Design review of the part built by this model. Coordinates are the model's own, in mm. A direction names the side the tool comes from. Coordinates: 2 decimals unless noted, no trailing zeros. Write each loop counter-clockwise with the first axis right and the second up, starting at its lowest first coordinate (ties: lowest second). Pieces come first, ordered by that corner, then holes.
Q1. To check wall thickness, follow probe 1 along X at (y, z) = (-20, -19.5); probe 2 along Z at (x, y) = (39, -14.75); probe 3 along Y at (x, z) = (41, -9.75). State the ranges of each line that lie inside material, in increasing order.
Q2. Add section D-D, the plane z = -6.25. Give the boundary of the cut face in (x, y).
Q3. Add section C-C, the plane y = -5.25. Give the boundary of the cut face in (x, z), plus the area to 3 significant figures.
Q4. Add section B-B, the plane z = -14.5. Give the boundary of the cut face in (x, y).
Q5. Clearance check with flat-ended pins moving along their axes: pin 1 Ø3 at (x, z) = (41.5, -11.5) entering from -Y; pin 2 Ø6.5 at (x, y) = (46.5, -16.5) entering from -Z; pin 3 Ø3 at (x, z) = (41.5, -11.5) entering from +Y. State where each tip first meets the part, or that it passes through.
Q6. Add section A-A, the plane y = -13.5. Give the boundary of the cut face in (x, z), plus the area to 3 significant figures.
Q7. Machinability: for faces 1 (the face through (44, -6.903, -13)), 2 (the face through (44, -14, -7.729)), 3 (the face through (44, -20.663, -13)), 4 (the face through (44, -14, -17.984)), 5 (the face through (18, 0, -14)), which of the approach directions +Z, -Z, +X, -X, +Y, -Y give a long, thin tool a straight path to every point of the face, cutting with its end or side? Answer none if there is none.
from build123d import *

# Parameters (mm, degrees)
F0_W     = 37.3699069023
F0_H     = 28.7381336093
F1_DEPTH = 25.4
F4_W     = 13.7605443597
F4_H     = 10.2546699345
F5_DEPTH = 12.7


# Not quite as in the source:
# - the program builds the solid bodies; features that only make, move or delete a surface that nothing else refers to are left out


with BuildPart() as f1:
    # F0 (on Front) → F1 (new body)
    with BuildSketch(Plane.XZ):
        with Locations((18.6849534512, -14.3690668046)):
            Rectangle(F0_W, F0_H)
    extrude(amount=F1_DEPTH)

    # F4 (on face) → F5 (join)
    with BuildSketch(Plane.YZ.offset(37.3699069023)):
        with Locations((-13.7830860913, -12.8563437611)):
            Rectangle(F4_W, F4_H)
    extrude(amount=F5_DEPTH)


solid = f1.part
Here are the results:
1. probe 1: x = 0 to 37.37
1. probe 2: z = -17.98 to -7.73
1. probe 3: y = -20.66 to -6.9
2. outline: (0, -25.4) - (37.37, -25.4) - (37.37, 0) - (0, 0) - close
3. outline: (0, -28.74) - (37.37, -28.74) - (37.37, 0) - (0, 0) - close
3. area: 1,070 mm2
4. outline: (0, -25.4) - (37.37, -25.4) - (37.37, -20.66) - (50.07, -20.66) - (50.07, -6.9) - (37.37, -6.9) - (37.37, 0) - (0, 0) - close
5. pin 1: stops at y = -20.66
5. pin 2: stops at z = -17.98
5. pin 3: stops at y = -6.9
6. outline: (0, -28.74) - (37.37, -28.74) - (37.37, -17.98) - (50.07, -17.98) - (50.07, -7.73) - (37.37, -7.73) - (37.37, 0) - (0, 0) - close
6. area: 1,200 mm2
7. face 1: +Z, -Z, +X, +Y
7. face 2: +Z, +X, +Y, -Y
7. face 3: +Z, -Z, +X, -Y
7. face 4: -Z, +X, +Y, -Y
7. face 5: +Z, -Z, +X, -X, +Y
